Input: part model. Units: mm. Frame: model coordinates. Coordinates: 2 decimals unless noted, no trailing zeros. Order: outer loops, then holes, each group sorted by start corner. A loop starts at its lowest first (then second) coordinate and runs counter-clockwise, first axis right, second up. Notation, with made-up numbers: M 84.5,73 L 97.5,73 A25 ccw 97.5,90 Z; hole C -5,-37 d3. An arc over 180 degrees is marked long. Answer in a Markdown table with one row per item.
from build123d import *

# Parameters (mm, degrees)
BOSS_EXTRUDE1_DEPTH      = 2.2
BOSS_EXTRUDE2_DEPTH      = 4.4
BOSS_EXTRUDE2_DEPTH_BACK = 2
SKETCH1_3_R              = 1.1


with BuildPart() as part:
    # Sketch1 → Boss-Extrude1 (new body)
    with BuildSketch(Plane(origin=(0, 0, 0), x_dir=(1, 0, 0), z_dir=(0, 1, 0))):
        with BuildLine():
            Line((5.523587939, -1.389168628), (5.523587939, -0.589168628))
            Line((5.523587939, -0.589168628), (0.373516405, 1.03464269))
            ThreePointArc((0.373516405, 1.03464269), (0.330776379, 1.049088646), (0.28747994, 1.061769883))
            Line((0.28747994, 1.061769883), (-1.533917496, 1.636054289))
            add(Edge.make_bspline(
                [(-3, 0.587196294), (-2.993093164, 1.205023593), (-2.177968287, 1.839122723), (-1.533917496, 1.636054289)],
                knots=[0, 0, 0, 0, 1, 1, 1, 1], degree=3))
            Line((-3, 0.587196294), (-3, 0.08639369))
            ThreePointArc((-3, 0.08639369), (-2.85, -0.173413931), (-2.55, -0.173413931))
            Line((-2.55, -0.173413931), (-1.95, 0.17299623))
            ThreePointArc((-1.95, 0.17299623), (-1.65, 0.17299623), (-1.5, -0.086811391))
            Line((-1.5, -0.086811391), (-1.5, -0.2))
            ThreePointArc((-1.5, -0.2), (-1.148528137, -1.048528137), (-0.3, -1.4))
            Line((-0.3, -1.4), (0, -1.4))
            add(Edge.make_bspline(
                [(5.523587939, -1.389168628), (5.523587939, -1.655644582), (5.31087633, -1.80182616), (4.791580785, -1.773367747), (4.77273176, -1.59674075), (3.415135688, -1.368008507), (2.1, -1.4), (0, -1.4)],
                knots=[0, 0, 0, 0, 0.200930821, 0.262112326, 0.572959193, 0.650633546, 1, 1, 1, 1], degree=3))
        make_face()
    extrude(amount=BOSS_EXTRUDE1_DEPTH)

    # Sketch1<3> → Boss-Extrude2 (add, two sides: drawn at the far end of the back side and taken through both)
    with BuildSketch(Plane(origin=(0, 0, 0), x_dir=(1, 0, 0), z_dir=(0, 1, 0)).offset(-BOSS_EXTRUDE2_DEPTH_BACK)):
        with Locations(Location((0, 0, 0), (0, 0, 270))):
            Circle(SKETCH1_3_R)
    extrude(amount=BOSS_EXTRUDE2_DEPTH + BOSS_EXTRUDE2_DEPTH_BACK)


solid = part.part
1) Cut plane A-A, the plane z = 0.8. Output: boundary loops of the cut face in (x, y), and give its area (3 significant figures).
Resolved:
| item | result |
|---|---|
| outline | M -1.34,0 L -0.75,0 L -0.75,-2 L 0.75,-2 L 0.75,0 L 5.52,0 L 5.52,2.2 L 0.75,2.2 L 0.75,4.4 L -0.75,4.4 L -0.75,2.2 L -1.34,2.2 Z |
| area | 21.4 mm2 |
2) Material intervals for probe 1 along Y at (x, z) = (5.25, 0.8); probe 2 along Z at (x, y) = (3.5, 1.75); probe 3 along X at (y, z) = (-1, -0.95), sorted ascending.
Resolved:
| item | result |
|---|---|
| probe 1 | y = 0 to 2.2 |
| probe 2 | z = -0.05 to 1.42 |
| probe 3 | x = -0.55 to 0.55 |
3) Cut plane B-B, the plane x = -1. Output: boundary loops of the cut face in (y, z), and give its area (3 significant figures).
Resolved:
| item | result |
|---|---|
| outline | M -2,-0.46 L 0,-0.46 L 0,-1.47 L 2.2,-1.47 L 2.2,-0.46 L 4.4,-0.46 L 4.4,0.46 L 2.2,0.46 L 2.2,1.17 L 0,1.17 L 0,0.46 L -2,0.46 Z |
| area | 9.66 mm2 |
4) Contact query for flat-ended pins moving along their axis: pin 1 (2 mm diameter, centred on x = 1, y = 3, fed in from -Z); pin 2 (1.5 mm diameter, centred on x = 0, y = 2.5, fed in from -Z). Output: stop coordinate, or through.
Resolved:
| item | result |
|---|---|
| pin 1 | stops at z = -1.1 |
| pin 2 | stops at z = -1.37 |
5) Mould query, pull axis Z, two halves, no side actions, for faces 1 (the face through (1.2, 2.2, 0.4)), 2 (the face through (-1.158, 1.085, 1.039)), 3 (the face through (-0.61, 1.085, -1.345)). Classes: +Z half, -Z half, draft (parallel to the pull), parting line (faces both ways), or undercut.
Resolved:
| item | result |
|---|---|
| face 1 | draft |
| face 2 | +Z half |
| face 3 | -Z half |
6) Cut plane C-C, the plane y = -0.25. Output: boundary loops of the cut face in (x, z), and give its area (3 significant figures).
Resolved:
| item | result |
|---|---|
| outline | C 0,0 d2.2 |
| area | 3.80 mm2 |
